Verification items for the finished model (mm, model axes). A direction names the side the tool comes from. Coordinates: 2 decimals unless noted, no trailing zeros. Write each loop counter-clockwise with the first axis right and the second up, starting at its lowest first coordinate (ties: lowest second). Pieces come first, ordered by that corner, then holes. Notation, with made-up numbers: M 15.25,19 L 32.25,19 A32 ccw 32.25,46 Z; hole C -18.5,-12 d7. An arc over 180 degrees is marked long. Answer in a Markdown table with one row per item.
from build123d import *

# Parameters (mm, degrees)
F1_DEPTH = 6
F0_W     = 20.403712
F0_H     = 20
F2_DEPTH = 5


with BuildPart() as f1:
    # F0 (on Top) → F1 (new body)
    with BuildSketch(Plane.XY):
        Polygon((-1.160592, 9.762301), (-14.150973, 17.262301), (-14.150973, 2.262301), align=None)
    extrude(amount=F1_DEPTH)

    # F0 (on Top) → F2 (join)
    with BuildSketch(Plane.XY):
        with Locations((-8.199221, 10)):
            Rectangle(F0_W, F0_H)
        Polygon((-14.150973, 2.262301), (-14.150973, 17.262301), (-1.160592, 9.762301), align=None, mode=Mode.SUBTRACT)
    extrude(amount=F2_DEPTH)


solid = f1.part
1) Tool access check on faces 4 (the face through (-7.565, 13.46, 5.493)), 5 (the face through (-7.75, 5.96, 5.49)), 6 (the face through (-18.401, 10, 2)). Record the directions out of +Z, -Z, +X, -X, +Y, -Y that give a thin tool (end or side, any length) a straight path to the whole face; none if there is none.
Response values:
| item | result |
|---|---|
| face 4 | +Z, +X, +Y |
| face 5 | +Z, +X, -Y |
| face 6 | +Z, -Z, -X, +Y, -Y |
2) Thickness scan on L1, parallel to Z at x = -4.25, y = 5.5; L2, parallel to Y at x = -12, z = 5.55; L3, parallel to X at y = 10, z = 5.8. Record the ranges inside material, lowest first. Write a range as [from, to].
Response values:
| item | result |
|---|---|
| L1 | z = [0, 5] |
| L2 | y = [3.5, 16.02] |
| L3 | x = [-14.15, -1.57] |
3) Release check for a two-part mould opening along X. For faces 1 (the face through (2.003, 10, 2)), 2 (the face through (-14.151, 9.9, 5.5)), 3 (the face through (-8, 10, 0)) record: +X half, -X half, draft (parallel to the pull), parting line (faces both ways), or undercut.
Response values:
| item | result |
|---|---|
| face 1 | +X half |
| face 2 | -X half |
| face 3 | draft |
4) Sectioned sample at B-B (y = 16). Record the cut outline in (x, z), then the cut area to 3 significant figures.
Response values:
| item | result |
|---|---|
| outline | M -18.4,0 L 2,0 L 2,5 L -11.96,5 L -11.96,6 L -14.15,6 L -14.15,5 L -18.4,5 Z |
| area | 104 mm² |
5) Sectioned sample at C-C (x = -16.25). Record the cut outline in (y, z), then the cut area to 3 significant figures.
Response values:
| item | result |
|---|---|
| outline | M 0,0 L 20,0 L 20,5 L 0,5 Z |
| area | 100 mm² |
6) Depth check by flat-ended pin: pin 1 (0.8 mm diameter, centred on y = 13, z = 5.5, fed in from -X). Enter the tip coordinate at first touch or a pass-through.
Response values:
| item | result |
|---|---|
| pin 1 | stops at x = -14.15 |
7) Sectioned sample at A-A (x = -11.25). Record the cut outline in (y, z), then the cut area to 3 significant figures.
Response values:
| item | result |
|---|---|
| outline | M 0,0 L 20,0 L 20,5 L 15.59,5 L 15.59,6 L 3.94,6 L 3.94,5 L 0,5 Z |
| area | 112 mm² |
